```python
from build123d import *

# Parameters (mm, degrees)
SKETCH1_W           = 26.9494
SKETCH1_H           = 26.9494
BOSS_EXTRUDE1_DEPTH = 3.6322
SKETCH2_W           = 23.114
SKETCH2_H           = 21.336
BOSS_EXTRUDE2_DEPTH = 20.5486
SKETCH3_R           = 2.26691968
SKETCH3_W           = 3.044100844
SKETCH3_H           = 9.672621698
CUT_EXTRUDE1_DEPTH  = 5


with BuildPart() as part:
    # Sketch1 → Boss-Extrude1 (new body)
    with BuildSketch(Plane(origin=(0, 0, 0), x_dir=(1, 0, 0), z_dir=(0, 1, 0))):
        with Locations((13.4747, 13.4747)):
            Rectangle(SKETCH1_W, SKETCH1_H)
    extrude(amount=BOSS_EXTRUDE1_DEPTH)

    # Sketch2 → Boss-Extrude2 (add)
    with BuildSketch(Plane(origin=(0, 3.6322, 0), x_dir=(1, 0, 0), z_dir=(0, 1, 0))):
        with Locations((13.4747, 13.4747)):
            Rectangle(SKETCH2_W, SKETCH2_H)
    extrude(amount=BOSS_EXTRUDE2_DEPTH)

    # Sketch3 → Cut-Extrude1 (cut)
    with BuildSketch(Plane.XZ):
        with Locations(Location((13.4747, -19.796472905, 0), (0, 0, 270))):
            Circle(SKETCH3_R)
        with Locations((7.585585607, -9.270512148)):
            Rectangle(SKETCH3_W, SKETCH3_H)
        with Locations((19.363814393, -9.270512148)):
            Rectangle(SKETCH3_W, SKETCH3_H)
    extrude(amount=-CUT_EXTRUDE1_DEPTH, mode=Mode.SUBTRACT)


solid = part.part
```
For this review, take the finished solid that the model builds, in its own axes (mm). A direction names the side the tool comes from. Give positions to 0.01 mm unless a question says otherwise; leave off trailing zeros. Write each loop counter-clockwise with the first axis right and the second up, starting at its lowest first coordinate (ties: lowest second). Pieces come first, ordered by that corner, then holes.
Item 1: Wall thickness on probe 1 along X at (y, z) = (3, -7.25); probe 2 along Y at (x, z) = (20.25, -7); probe 3 along Z at (x, y) = (9, 3.25): over which ranges is each line inside the solid? List them lowest first.
Item 2: Take a section at C-C (x = 19.5). Give the boundary of the cut face in (y, z), and give its area (3 significant figures).
Item 3: The part is to be moulded in two halves that separate along X. For faces 1 (the face through (19, 2, -4.434)), 2 (the face through (25.032, 14, -13)), 3 (the face through (13, 0, -14)), 4 (the face through (8, 2, -14.107)), say which applies: +X half, -X half, draft (parallel to the pull), parting line (faces both ways), or undercut.
Item 4: Take a section at B-B (y = 4). Give the boundary of the cut face in (x, z).
Item 5: Insertion check: P1, Ø2, axis at y = 11.5, z = -7.5, coming from the -X side; P2, Ø1.5, axis at y = 5, z = -19.5, coming from the +X side; P3, Ø2.5, axis at x = 13.47, z = -19.8, coming from the -Y side. Each pin has a flat end and moves straight along its axis. Give the tip position at first contact, or say it passes through.
Item 6: Take a section at A-A (z = -7). Give the boundary of the cut face in (x, y).
Item 7: Machinability: for faces 5 (the face through (9.108, 2, -9)), 6 (the face through (1.918, 14, -13)), 7 (the face through (13, 14, -2.807)), 8 (the face through (13, 14, -24.143)), 9 (the face through (0, 2, -13)), which of the approach directions +Z, -Z, +X, -X, +Y, -Y give a long, thin tool a straight path to every point of the face, cutting with its end or side? Answer none if there is none.
Item 8: Take a section at D-D (y = 14.5). Give the boundary of the cut face in (x, z), and give its area (3 significant figures).
Established:
1. probe 1: x = 0 to 6.06, 9.11 to 17.84, 20.89 to 26.95
1. probe 2: y = 5 to 24.18
1. probe 3: z = -26.95 to -14.11, -4.43 to 0
2. outline: (0, -26.95) - (3.63, -26.95) - (3.63, -24.14) - (24.18, -24.14) - (24.18, -2.81) - (3.63, -2.81) - (3.63, 0) - (0, 0) - (0, -4.43) - (5, -4.43) - (5, -14.11) - (0, -14.11) - close
2. area: 488 mm2
3. face 1: undercut
3. face 2: +X half
3. face 3: draft
3. face 4: undercut
4. outline: (1.92, -24.14) - (25.03, -24.14) - (25.03, -2.81) - (1.92, -2.81) - close; hole (6.06, -14.11) - (9.11, -14.11) - (9.11, -4.43) - (6.06, -4.43) - close; hole circle Ø4.53 at (13.47, -19.8); hole (17.84, -14.11) - (20.89, -14.11) - (20.89, -4.43) - (17.84, -4.43) - close
5. P1: stops at x = 1.92
5. P2: stops at x = 25.03
5. P3: stops at y = 5
6. outline: (0, 0) - (6.06, 0) - (6.06, 5) - (9.11, 5) - (9.11, 0) - (17.84, 0) - (17.84, 5) - (20.89, 5) - (20.89, 0) - (26.95, 0) - (26.95, 3.63) - (25.03, 3.63) - (25.03, 24.18) - (1.92, 24.18) - (1.92, 3.63) - (0, 3.63) - close
7. face 5: -Y
7. face 6: +Z, -Z, -X, +Y
7. face 7: +Z, +X, -X, +Y
7. face 8: -Z, +X, -X, +Y
7. face 9: +Z, -Z, -X, +Y, -Y
8. outline: (1.92, -24.14) - (25.03, -24.14) - (25.03, -2.81) - (1.92, -2.81) - close
8. area: 493 mm2
